```python
from build123d import *

# Parameters (mm, degrees)
BOSS_EXTRUDE1_DEPTH = 11
CHAMFER1_SIZE       = 3
SKETCH2_R           = 1.5
CUT_EXTRUDE1_DEPTH  = 39.050256569
CUT_EXTRUDE2_DEPTH  = 41.047746816
FILLET1_R           = 1


with BuildPart() as part:
    # Sketch1 → Boss-Extrude1 (new body)
    with BuildSketch(Plane.XY):
        Polygon((-26.955, 0), (-17.955, 0), (-17.955, 24.5), (17.955, 24.5), (17.955, 0), (26.955, 0), (26.955, 3), (20.955, 3), (20.955, 27.5), (-20.955, 27.5), (-20.955, 3), (-26.955, 3), align=None)
    extrude(amount=BOSS_EXTRUDE1_DEPTH)

    # Chamfer1
    chamfer1_edges = [part.edges().sort_by_distance(p)[0] for p in [
        (-26.955, 1.5, 0),
        (26.955, 1.5, 0),
        (26.955, 1.5, 11),
        (-26.955, 1.5, 11),
    ]]
    chamfer(chamfer1_edges, length=CHAMFER1_SIZE)

    # Sketch2 → Cut-Extrude1 (cut, through all)
    with BuildSketch(Plane(origin=(0, 3, 0), x_dir=(1, 0, 0), z_dir=(0, 1, 0))):
        with Locations(Location((-23.955, -5.5, 0), (0, 0, 180))):
            Circle(SKETCH2_R)
        with Locations((23.955, -5.5)):
            Circle(SKETCH2_R)
    extrude(amount=-CUT_EXTRUDE1_DEPTH, mode=Mode.SUBTRACT)

    # Sketch3 → Cut-Extrude2 (cut, through all)
    with BuildSketch(Plane.XY.offset(11)):
        with BuildLine():
            Line((-14.305, 26.15), (-10.105, 26.15))
            ThreePointArc((-10.105, 26.15), (-8.455, 24.5), (-10.105, 22.85))
            Line((-10.105, 22.85), (-14.305, 22.85))
            ThreePointArc((-14.305, 22.85), (-15.955, 24.5), (-14.305, 26.15))
        make_face()
    extrude(amount=-CUT_EXTRUDE2_DEPTH, mode=Mode.SUBTRACT)

    # Fillet1
    fillet1_edges = [part.edges().sort_by_distance(p)[0] for p in [
        (-15.955, 24.5, 5.5),
        (-8.455, 24.5, 5.5),
    ]]
    fillet(fillet1_edges, radius=FILLET1_R)


solid = part.part
```
For this review, take the finished solid that the model builds, in its own axes (mm). A direction names the side the tool comes from. Coordinates: 2 decimals unless noted, no trailing zeros. Order: outer loops, then holes, each group sorted by start corner. A loop starts at its lowest first (then second) coordinate and runs counter-clockwise, first axis right, second up. Notation, with made-up numbers: (8, -5.75) - (19, -5.75) arc R15 ccw to (19, 17.25) - close; hole circle Ø3 at (46, 25.5). An arc over 180 degrees is marked (long way). Answer as a JSON object with one key per item and string values. Group by question number.
1. We need section C-C on x = 0. State the section outline as (y, z) points, then the cut area to 3 significant figures.
2. For faces 4 (the flat face through (20.955, 15, 5)), 5 (the flat face through (-20.955, 15, 5)), 6 (the flat face through (17.955, 12, 5)), list the 3-axis set-ups (+Z, -Z, +X, -X, +Y, -Y) from which the entire face can be reached by the end or side of a thin tool; tool diameter is ignored.
3. For probe 1 along X at (y, z) = (16.25, 4.75) (3 decimals); probe 2 along Y at (x, z) = (0.5, 6.5); probe 3 along Y at (x, z) = (-11.5, 8.5), list the stretches that pass through material, from the lowest coordinate up.
4. We need section D-D on z = 1. State the section outline as (x, y) points (3 decimals).
5. The part is to be moulded in two halves that separate along X. For faces 1 (the cylindrical face through (-9.2, 25.88, 5.58)), 2 (the flat face through (22, 0, 5)), 3 (the flat face through (26.955, 1, 5)), say which applies: pulls with the +X half, pulls with the -X half, needs draft (parallel to the pull), parting line crosses it, or undercut.
6. Clearance check with flat-ended pins moving along their axes: P1, Ø8, axis at x = -1.5, y = 23, coming from the -Z side; P2, Ø5.5, axis at y = 10.5, z = 8, coming from the -X side (3 decimals); P3, Ø5.5, axis at y = 20.5, z = 3.5, coming from the +X side (3 decimals); P4, Ø1.3, axis at x = -12.5, z = 3, coming from the -Y side. State where each tip first meets the part, or that it passes through.
7. We need section A-A on y = 11. State the section outline as (x, z) points (3 decimals), then the cut area to 3 significant figures.
8. We need section B-B on z = 5.5. State the section outline as (x, y) points (3 decimals), then the cut area to 3 significant figures.
Final values:
{
 "1": {"outline": "(24.5, 0) - (27.5, 0) - (27.5, 11) - (24.5, 11) - close", "area": "33.0 mm²"},
 "2": {"face 4": "+Z, -Z, +X, +Y", "face 5": "+Z, -Z, -X, +Y", "face 6": "+Z, -Z, -Y"},
 "3": {"probe 1": "-20.955 to -17.955, 17.955 to 20.955", "probe 2": "24.5 to 27.5", "probe 3": "26.15 to 27.5"},
 "4": {"outline": "(-24.955, 0) - (-17.955, 0) - (-17.955, 24.5) - (-16.759, 24.5) arc R1 ccw to (-15.833, 25.123) arc R1.65 cw to (-14.305, 26.15) - (-10.105, 26.15) arc R1.65 cw to (-8.577, 25.123) arc R1 ccw to (-7.651, 24.5) - (17.955, 24.5) - (17.955, 0) - (24.955, 0) - (24.955, 3) - (20.955, 3) - (20.955, 27.5) - (-20.955, 27.5) - (-20.955, 3) - (-24.955, 3) - close"},
 "5": {"face 1": "undercut", "face 2": "needs draft", "face 3": "pulls with the +X half"},
 "6": {"P1": "z = 0", "P2": "x = -20.955", "P3": "x = 20.955", "P4": "y = 26.15"},
 "7": {"outline": "(-20.955, 0) - (-17.955, 0) - (-17.955, 11) - (-20.955, 11) - close; (17.955, 0) - (20.955, 0) - (20.955, 11) - (17.955, 11) - close", "area": "66.0 mm²"},
 "8": {"outline": "(-26.955, 0) - (-25.455, 0) - (-25.455, 3) - (-26.955, 3) - close; (-22.455, 0) - (-17.955, 0) - (-17.955, 24.5) - (-16.759, 24.5) arc R1 ccw to (-15.833, 25.123) arc R1.65 cw to (-14.305, 26.15) - (-10.105, 26.15) arc R1.65 cw to (-8.577, 25.123) arc R1 ccw to (-7.651, 24.5) - (17.955, 24.5) - (17.955, 0) - (22.455, 0) - (22.455, 3) - (20.955, 3) - (20.955, 27.5) - (-20.955, 27.5) - (-20.955, 3) - (-22.455, 3) - close; (25.455, 0) - (26.955, 0) - (26.955, 3) - (25.455, 3) - close", "area": "279 mm²"}
}
